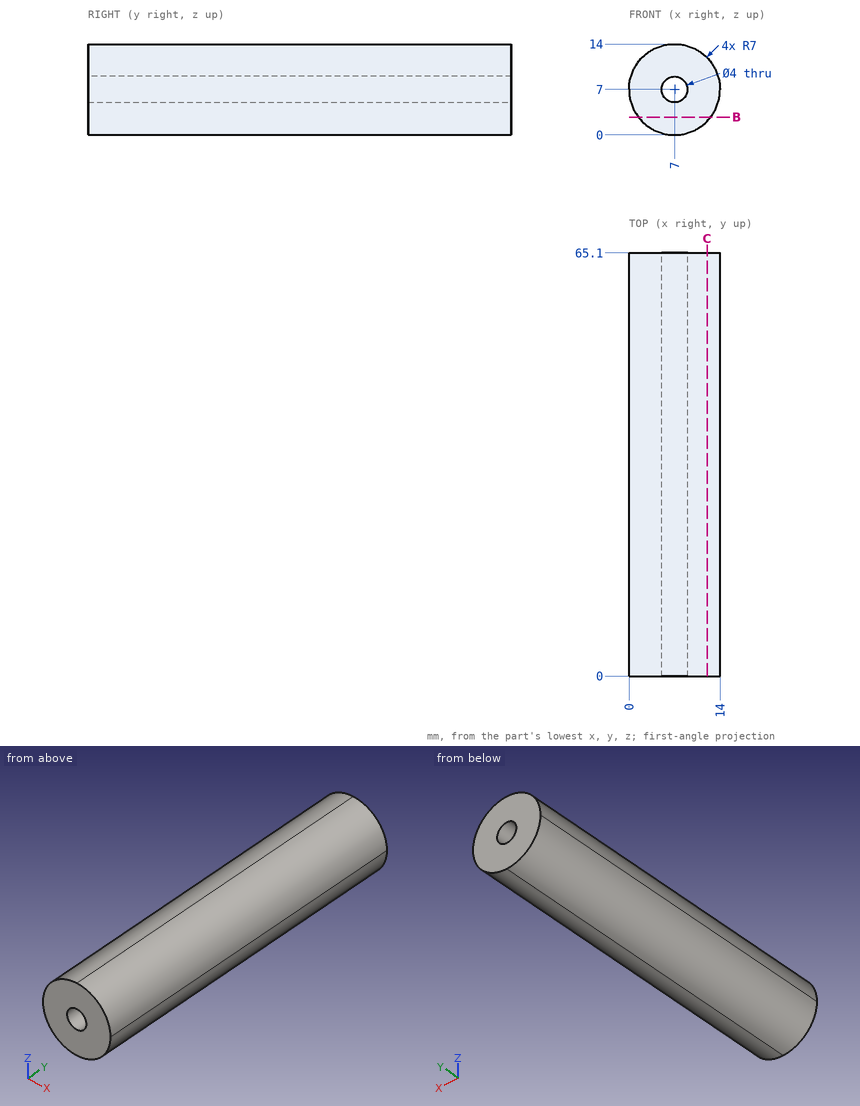
Check sheet for the drawn part. Datum: minimum x, y, z corner. Units: mm. Coordinates: 2 decimals unless noted, no trailing zeros. Loops run counter-clockwise (first coordinate to the right, second up) from the corner with the lowest first, then second, coordinate; pieces in that order, holes last. Notation, with made-up numbers: (55, 56.25) -> (67, 56.25) arc R20 ccw to (67, 94.25) -> close; hole circle Ø9 at (68, 41.5). An arc over 180 degrees is marked (long way). Write each question's results on one line, items separated by ' | '.
Item 1: Section check B-B, the plane z = 2.75. Enter the section's corners in (x, y), plus the area to 3 significant figures.
Found:
outline: (1.44, 0) -> (12.56, 0) -> (12.56, 65.1) -> (1.44, 65.1) -> close | area: 724 mm2
Item 2: Material ranges on L1, parallel to X at y = 24, z = 7; L2, parallel to Z at x = 6.5, y = 49; L3, parallel to Z at x = 6, y = 20, recorded low to high.
Found:
L1: x = 0 to 5, 9 to 14 | L2: z = 0.02 to 5.06, 8.94 to 13.98 | L3: z = 0.07 to 5.27, 8.73 to 13.93
Item 3: Gauge pin test, flat ends, axial feed: pin 1 (4 mm diameter, centred on x = 9, y = 51, fed in from -Z); pin 2 (1 mm diameter, centred on y = 25, z = 5, fed in from +X). Record the tip position at first contact, or that the pin passes through.
Found:
pin 1: stops at z = 0 | pin 2: stops at x = 13.84
Item 4: Section check C-C, the plane x = 12. Enter the section's corners in (y, z), plus the area to 3 significant figures.
Found:
outline: (0, 2.1) -> (65.1, 2.1) -> (65.1, 11.9) -> (0, 11.9) -> close | area: 638 mm2
